Autodesk Inventor part; units mm, degrees
ref_plane "YZ Plane" through (0, 0, 0) normal (1, 0, 0) x (0, 1, 0)
ref_plane "XZ Plane" through (0, 0, 0) normal (0, 1, 0) x (-1, 0, 0)
ref_plane "XY Plane" through (0, 0, 0) normal (0, 0, 1) x (1, 0, 0)
sketch "Sketch1" plane through (0, 0, 0) normal (0, 0, 1) x (1, 0, 0)
  line L0 (-14.5, 2.75) -> (14.5, 2.75)
  line L1 (14.5, 2.75) -> (14.5, -2.75)
  line L2 (14.5, -2.75) -> (-14.5, -2.75)
  line L3 (-14.5, -2.75) -> (-14.5, 2.75)
  line L4 (-14.5, 2.75) -> (14.5, -2.75) construction
  line L5 (14.5, 2.75) -> (-14.5, -2.75) construction
  point P0 (0, 0)
  dimension "d0" = 29
  dimension "d1" = 5.5
extrude "Extrusion1" add sketch "Sketch1" along normal blind 17
sketch "Sketch2" plane through (-14.5, 2.75, 0) normal (0, 1, 0) x (1, 0, 0)
  circle A0 centre (13.5, 0.5) radius 6.5
  line L0 (0, 0) -> (0, -17)
  line L1 (29, -17) -> (0, -17)
  point P0 (19.9809, 0.0015)
  point P1 (7.0191, 0.0015)
  dimension "d5" = 13
  dimension "d6" = 13.5
  dimension "d10" = 17.5
extrude "Extrusion2" cut sketch "Sketch2" against normal through all
sketch "Sketch3" plane through (0, 0, 0) normal (0, 0, -1) x (-1, 0, 0)
  circle A0 centre (11, 0) radius 2.25
  line L0 (7.4807, -2.75) -> (14.5, -2.75)
  line L1 (14.5, -2.75) -> (14.5, 2.75)
  circle A1 centre (-9, 0) radius 2.25
  line L2 (-14.5, -2.75) -> (-5.4807, -2.75)
  point P0 (0, 0)
  dimension "d11" = 4.5
  dimension "d12" = 2.75
  dimension "d13" = 3.5
  dimension "d14" = 4.5
  dimension "d15" = 20
  dimension "d16" = 2.75
hole "Hole1" at (9, 0, 0) at (-11, 0, 0) direction (0, 0, 1) diameter 4.5 end through all
fillet "Fillet1" radius 2 2 edges at (-14.5, 0, 17) (14.5, 0, 17)
properties part number "CarroXY - HotendFrente"
The listing builds one solid part. Answer for the finished solid, in the listing's coordinates (mm). Give positions to 0.01 mm unless a question says otherwise; leave off trailing zeros. Order: outer loops, then holes, each group sorted by start corner. A loop starts at its lowest first (then second) coordinate and runs counter-clockwise, first axis right, second up. Notation, with made-up numbers: M 4.5,53.25 L 38.5,53.25 A20 cw 38.5,77.25 Z; hole C -29,26.5 d2. An arc over 180 degrees is marked long. Put each result on its own line as item: value. Start each with the question number.
Item 1: The part is cut by section A-A, the plane x = 9. Determine the outline of the cut face in (y, z), and give its area (3 significant figures).
Item 2: For a pull along Y with two mould halves and no side action, classify faces 1 (the face through (-13.23, -0.29, 8.62)), 2 (the face through (0, 2.75, 8)), 3 (the face through (-1, 0, 6)) as +Y half, -Y half, draft (parallel to the pull), parting line (faces both ways), or undercut.
Item 3: The part is cut by section C-C, the plane z = 7.75. Determine the outline of the cut face in (x, y), and give its area (3 significant figures).
Item 4: Find the intervals of material crossed by line 1 along X through (y, z) = (0, 7.5); line 2 along X through (y, z) = (1.6, 8.5); line 3 along X through (y, z) = (0, 4), in increasing order.
Item 5: The part is cut by section D-D, the plane x = 1.5. Determine the outline of the cut face in (y, z), and give its area (4 significant figures).
Item 6: The part is cut by section B-B, the plane y = -0.5. Determine the outline of the cut face in (x, z), and give its area (3 significant figures).
Answer key:
1. outline: M -2.75,0 L -2.25,0 L -2.25,17 L -2.75,17 Z; M 2.25,0 L 2.75,0 L 2.75,17 L 2.25,17 Z
1. area: 17.0 mm²
2. face 1: undercut
2. face 2: +Y half
2. face 3: draft
3. outline: M -14.5,-2.75 L 14.5,-2.75 L 14.5,2.75 L -14.5,2.75 Z; hole C -11,0 d4.5; hole C 9,0 d4.5
3. area: 128 mm²
4. line 1: x = -14.5 to -13.25, -8.75 to 6.75, 11.25 to 14.5
4. line 2: x = -14.5 to -12.58, -9.42 to 7.42, 10.58 to 14.5
4. line 3: x = -14.5 to -13.25, -8.75 to -5.69, 3.69 to 6.75, 11.25 to 14.5
5. outline: M -2.75,5.5 L 2.75,5.5 L 2.75,17 L -2.75,17 Z
5. area: 63.25 mm²
6. outline: M -14.5,0 L -13.19,0 L -13.19,16.88 A2 ccw -14.5,15 Z; M -8.81,0 L -7.48,0 A6.5 cw 5.48,0 L 6.81,0 L 6.81,17 L -8.81,17 Z; M 11.19,0 L 14.5,0 L 14.5,15 A2 ccw 12.5,17 L 11.19,17 Z
6. area: 282 mm²
